Could you check a few things on this model? Use its own coordinates, in mm. A direction names the side the tool comes from. Give positions to 0.01 mm unless a question says otherwise; leave off trailing zeros. Write each loop counter-clockwise with the first axis right and the second up, starting at its lowest first coordinate (ties: lowest second). Pieces come first, ordered by that corner, then holes. Notation, with made-up numbers: (-14, 43) - (26, 43) arc R25 cw to (26, 69) - close; hole circle Ø4 at (22, 15). An arc over 180 degrees is marked (long way). Answer as a JSON object with one key per item and string values. Group by question number.
Autodesk Inventor part; units mm, degrees
ref_plane "YZ Plane" through (0, 0, 0) normal (1, 0, 0) x (0, 1, 0)
ref_plane "XZ Plane" through (0, 0, 0) normal (0, 1, 0) x (-1, 0, 0)
ref_plane "XY Plane" through (0, 0, 0) normal (0, 0, 1) x (1, 0, 0)
sketch "Sketch1" plane through (0, 0, 0) normal (0, 1, 0) x (-1, 0, 0)
  line L0 (0, 0) -> (0, -20)
  line L1 (0, -20) -> (-14.7721, -22.6047)
  line L2 (-14.7721, -22.6047) -> (-14.7721, -17.6047)
  line L3 (-14.7721, -17.6047) -> (-10.0737, -19.3148)
  line L4 (0, 0) -> (-14.7721, 2.6047)
  line L5 (-14.7721, 2.6047) -> (-14.7721, -2.3953)
  line L6 (-14.7721, -2.3953) -> (-10.0737, -0.6852)
  line L7 (-10.0737, -0.6852) -> (-10.0737, -19.3148)
  dimension "d0" = 20
  dimension "d1" = 15
  dimension "d2" = 100
  dimension "d3" = 5
  dimension "d4" = 5
  dimension "d5" = 70
  dimension "d6" = 15
  dimension "d7" = 5
  dimension "d8" = 5
extrude "Extrusion1" add sketch "Sketch1" along normal blind 20
sketch "Sketch2" plane through (0, 0, -20) normal (-1, 0, 0) x (0, 0, 1)
  line L0 (0, 0) -> (0, 20)
  line L1 (20, 0) -> (0, 0)
  line L2 (0, 0) -> (0, 20)
  line L3 (0, 20) -> (20, 20)
  line L4 (20, 20) -> (20, 0)
extrude "Extrusion2" add sketch "Sketch2" along normal blind 5
sketch "Sketch3" plane through (0, 0, -20) normal (0, 0, -1) x (-1, 0, 0)
  line L0 (5, 20) -> (5, 0)
  line L1 (5, 20) -> (5, 0)
  line L2 (5, 0) -> (5, 5)
  line L3 (5, 20) -> (5, 15)
  line L4 (5, 15) -> (2.4019, 16.5)
  line L5 (5, 15) -> (8, 15) construction
  line L6 (5, 5) -> (2.4019, 3.5)
  line L7 (2.4019, 3.5) -> (2.4019, 16.5)
  line L8 (5, 20) -> (-5, 20)
  line L9 (5, 15) -> (5, 5)
  point P0 (0, 0)
  point P1 (5, 5)
  dimension "d13" = 5
  dimension "d14" = 5
  dimension "d15" = 3
  dimension "d16" = 150
  dimension "d17" = 3
extrude "Extrusion3" cut sketch "Sketch3" against normal blind 50
equation "\"BendRadius\" = Thickness"
equation "\"BendReliefWidth\" = Thickness"
equation "\"BendReliefDepth\" = 0.5 * Thickness"
equation "\"CornerReliefSize\" = 4 * Thickness"
equation "\"MinimumRemnant\" = 2 * Thickness"
equation "\"TransitionRadius\" = BendRadius"
equation "\"JacobiRadiusSize\" = BendRadius"
equation "\"GapSize\" = Thickness"
properties part number "Part1x"
(1) I want a section at A-A, the plane y = 17. Please give me the cut outline in (x, z), and give its area (3 significant figures).
(2) For faces 1 (the flat face through (-2.402, 10, -10)), 2 (the flat face through (-2, 10, -20)), 3 (the flat face through (10.074, 10, -10)), 4 (the flat face through (-2, 10, 0)), which set-ups out of +Z, -Z, +X, -X, +Y, -Y let a thin tool reach every point of the face, with its end or its side?
(3) I want a section at D-D, the plane y = 4. Please give me the cut outline in (x, z).
(4) I need wall thicknesses on L1, parallel to X at y = 11.5, z = -15; L2, parallel to Z at x = 12.25, y = 5.75; L3, parallel to X at y = 18, z = -14.75. Which ranges of each line are inside material? Lowest first, please.
(5) Will these pins go through, and if not, where does the flat tip stop? P1, Ø3, axis at x = 5.5, y = 7.5, coming from the +Z side; P2, Ø2.5, axis at x = -1.5, y = 5.5, coming from the +Z side; P3, Ø1.5, axis at x = -2.5, y = 10, coming from the -Z side.
(6) I want a section at C-C, the plane z = -17. Please give me the cut outline in (x, y), and give its area (3 significant figures).
(7) If we mould it in two halves opening along Y, with no side actions, what happens to faces 5 (the flat face through (-3.72, 15.74, -10.14)), 6 (the flat face through (5, 0, -10)), 7 (the flat face through (-5, 18, -10))? For each: +Y half, -Y half, draft (parallel to the pull), parting line (faces both ways), or undercut.
(8) I want a section at B-B, the plane x = -3.25. Please give me the cut outline in (y, z), and give its area (3 significant figures).
Entries:
{
 "1": {"outline": "(-5, -20) - (0, -20) - (14.77, -22.6) - (14.77, -17.6) - (10.07, -19.31) - (10.07, -0.69) - (14.77, -2.4) - (14.77, 2.6) - (0, 0) - (-5, 0) - close", "area": "354 mm^2"},
 "2": {"face 1": "+Z, -Z", "face 2": "-Z, -X, +Y, -Y", "face 3": "+Y, -Y", "face 4": "+Z, -X, +Y, -Y"},
 "3": {"outline": "(-5, -20) - (-3.27, -20) - (-3.27, 0) - (-5, 0) - close; (-2.4, -20) - (0, -20) - (14.77, -22.6) - (14.77, -17.6) - (10.07, -19.31) - (10.07, -0.69) - (14.77, -2.4) - (14.77, 2.6) - (0, 0) - (-2.4, 0) - close"},
 "4": {"L1": "-2.4 to 10.07", "L2": "-22.16 to -18.52, -1.48 to 2.16", "L3": "-5 to 10.07"},
 "5": {"P1": "z = 1.23", "P2": "z = 0", "P3": "z = -20"},
 "6": {"outline": "(-5, 0) - (10.07, 0) - (10.07, 20) - (-5, 20) - (-5, 15) - (-2.4, 16.5) - (-2.4, 3.5) - (-5, 5) - close", "area": "272 mm^2"},
 "7": {"face 5": "undercut", "face 6": "-Y half", "face 7": "draft"},
 "8": {"outline": "(0, -20) - (3.99, -20) - (3.99, 0) - (0, 0) - close; (16.01, -20) - (20, -20) - (20, 0) - (16.01, 0) - close", "area": "160 mm^2"}
}
